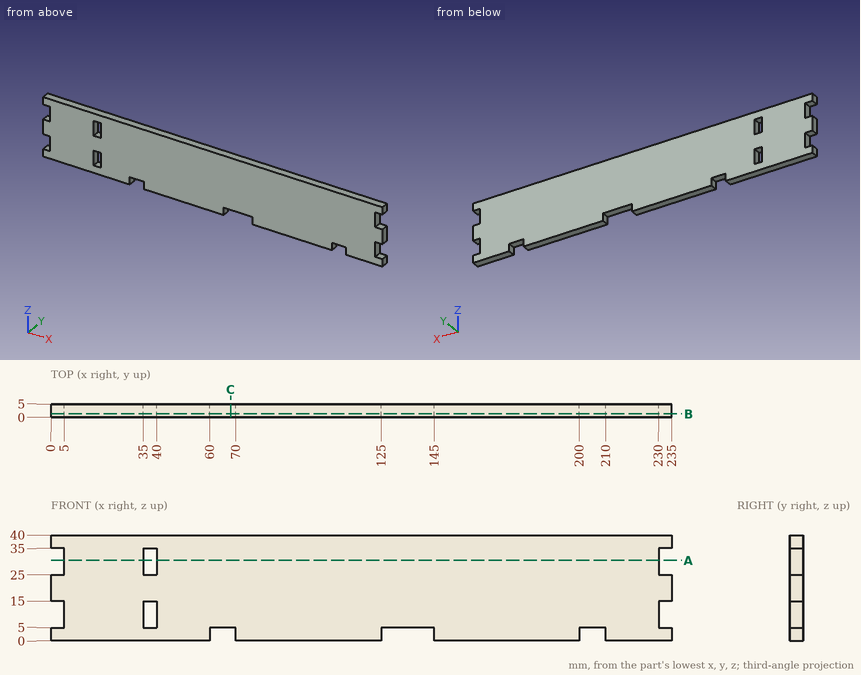
Can you work these out from the drawing? Everything is in mm from the part's minimum corner. Coordinates: 2 decimals unless noted, no trailing zeros. Loops run counter-clockwise (first coordinate to the right, second up) from the corner with the lowest first, then second, coordinate; pieces in that order, holes last.
1) Imagine slicing it at A-A on z = 30.5. List the corners of the cut face in (x, y) for me.
2) Imagine slicing it at C-C on x = 68. List the corners of the cut face in (y, z) for me, plus the area to 3 significant figures.
3) For pin 1 (2.5 mm diameter, centred on y = 3.5, z = 28.5, fed in from -X); pin 2 (1.5 mm diameter, centred on y = 2.5, z = 9.5, fed in from +X), each with a flat end and sliding along its axis, tell me the tip position at first contact or that it passes through.
4) Imagine slicing it at B-B on y = 1.25. State how many separate pieces and enclosed holes the cut face has, plus the area to 3 significant figures.
5) I need wall thicknesses on probe 1 along X at (y, z) = (4.6, 29.5); probe 2 along Z at (x, y) = (135, 3.8). Which ranges of each line are inside material? Lowest first, please.
Completed:
1. outline: (5, 0) - (35, 0) - (35, 5) - (5, 5) - close; (40, 0) - (230, 0) - (230, 5) - (40, 5) - close
2. outline: (0, 5) - (5, 5) - (5, 40) - (0, 40) - close
2. area: 175 mm2
3. pin 1: stops at x = 5
3. pin 2: stops at x = 230
4. separate pieces: 1
4. enclosed holes: 2
4. area: 8,900 mm2
5. probe 1: x = 5 to 35, 40 to 230
5. probe 2: z = 5 to 40
